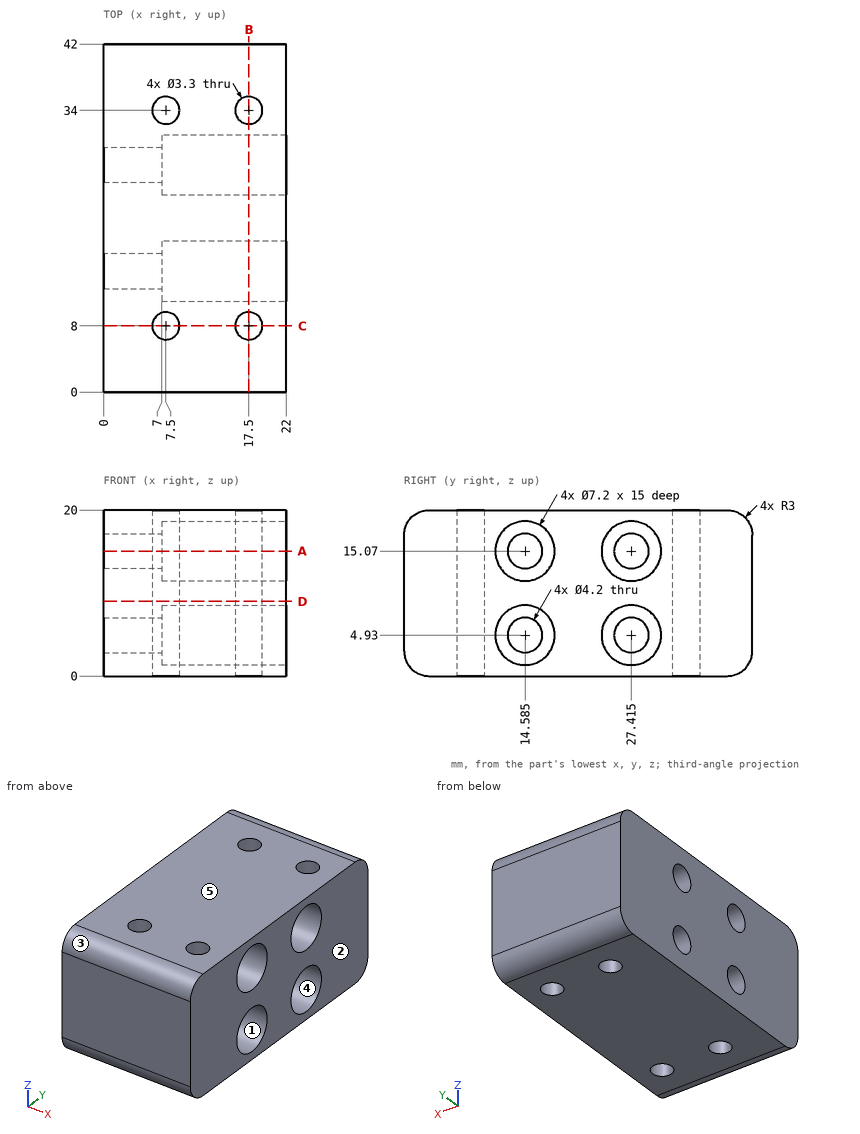
Answer from the drawing. Dimensions are ordinates in mm from the lowest x, y and z of the part. A direction names the side the tool comes from. Round coordinates to 2 decimals unless told otherwise and drop trailing zeros. Loops run counter-clockwise (first coordinate to the right, second up) from the corner with the lowest first, then second, coordinate; pieces in that order, holes last.
Q1. Section A-A on z = 15.07 is taken. Write down the section's boundary in (x, y) (3 decimals), and give its area (3 significant figures).
Q2. Each of these flat-tipped pins is pushed along its axis until it touches: pin 1 (6.5 mm diameter, centred on y = 14.585, z = 15.07, fed in from +X); pin 2 (1.5 mm diameter, centred on y = 14.5, z = 5.5, fed in from +X). Where does it stop, or does it pass through?
Q3. Consider probe 1 along Y at (x, z) = (3.5, 4.75); probe 2 along Z at (x, y) = (19.25, 14.5); probe 3 along Y at (x, z) = (3.25, 5.5). Determine where each line is inside the solid, lowest interval first.
Q4. Which of the six approach directions +Z, -Z, +X, -X, +Y, -Y give full straight-line access (tool end or side, diameter ignored) to the marked faces 4 and 5?
Q5. Section D-D on z = 9 is taken. Write down the section's boundary in (x, y), and give its area (3 significant figures).
Q6. Section C-C on y = 8 is taken. Write down the section's boundary in (x, z), and give its area (3 significant figures).
Q7. Determine the mould class of the marked faces 1, 2 and 3 for opening direction Z: released by +Z, released by -Z, zero draft, split by the parting line, or undercut.
Q8. Section B-B on x = 17.5 is taken. Write down the section's boundary in (y, z) (3 decimals).
Output:
1. outline: (0, 0) - (22, 0) - (22, 10.985) - (7, 10.985) - (7, 12.485) - (0, 12.485) - close; (0, 16.685) - (7, 16.685) - (7, 18.185) - (22, 18.185) - (22, 23.815) - (7, 23.815) - (7, 25.315) - (0, 25.315) - close; (0, 29.515) - (7, 29.515) - (7, 31.015) - (22, 31.015) - (22, 42) - (0, 42) - close; hole circle Ø3.3 at (7.5, 8); hole circle Ø3.3 at (7.5, 34); hole circle Ø3.3 at (17.5, 8); hole circle Ø3.3 at (17.5, 34)
1. area: 615 mm2
2. pin 1: stops at x = 7
2. pin 2: passes through
3. probe 1: y = 0 to 12.49, 16.68 to 25.32, 29.51 to 42
3. probe 2: z = 0 to 1.33, 8.53 to 11.47, 18.67 to 20
3. probe 3: y = 0 to 12.56, 16.61 to 25.39, 29.44 to 42
4. face 4: +X
4. face 5: +Z, +X, -X, +Y, -Y
5. outline: (0, 0) - (22, 0) - (22, 42) - (0, 42) - close; hole circle Ø3.3 at (7.5, 8); hole circle Ø3.3 at (7.5, 34); hole circle Ø3.3 at (17.5, 8); hole circle Ø3.3 at (17.5, 34)
5. area: 890 mm2
6. outline: (0, 0) - (5.85, 0) - (5.85, 20) - (0, 20) - close; (9.15, 0) - (15.85, 0) - (15.85, 20) - (9.15, 20) - close; (19.15, 0) - (22, 0) - (22, 20) - (19.15, 20) - close
6. area: 308 mm2
7. face 1: undercut
7. face 2: zero draft
7. face 3: released by +Z
8. outline: (0, 3) arc R3 ccw to (3, 0) - (6.35, 0) - (6.35, 20) - (3, 20) arc R3 ccw to (0, 17) - close; (9.65, 0) - (32.35, 0) - (32.35, 20) - (9.65, 20) - close; (35.65, 0) - (39, 0) arc R3 ccw to (42, 3) - (42, 17) arc R3 ccw to (39, 20) - (35.65, 20) - close; hole circle Ø7.2 at (14.585, 4.93); hole circle Ø7.2 at (14.585, 15.07); hole circle Ø7.2 at (27.415, 4.93); hole circle Ø7.2 at (27.415, 15.07)
